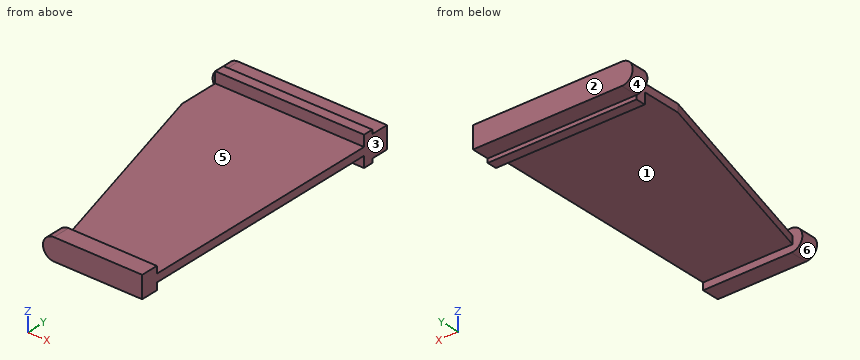
from build123d import *

# Parameters (mm, degrees)
BOSS_EXTRUDE1_DEPTH = 2.000000064
BOSS_EXTRUDE2_DEPTH = 4.4958
BOSS_EXTRUDE3_DEPTH = 4.4958
SKETCH4_W           = 38.1
SKETCH4_H           = 7.62
BOSS_EXTRUDE4_DEPTH = 2.54


with BuildPart() as part:
    # Sketch1 → Boss-Extrude1 (new body)
    with BuildSketch(Plane.XY):
        Polygon((0, 0), (-22.86, 0), (-38.1, 53.34), (-38.1, 66.04), (0, 66.04), align=None)
    extrude(amount=BOSS_EXTRUDE1_DEPTH)

    # Sketch2 → Boss-Extrude2 (add)
    with BuildSketch(Plane.XZ):
        with BuildLine():
            Line((0, -1.793999968), (-22.606, -1.793999968))
            ThreePointArc((-22.606, -1.793999968), (-25.4, 1.000000032), (-22.606, 3.794000032))
            Line((-22.606, 3.794000032), (0, 3.794000032))
            Line((0, 3.794000032), (0, -1.793999968))
        make_face()
    extrude(amount=BOSS_EXTRUDE2_DEPTH)

    # Sketch3 → Boss-Extrude3 (add)
    with BuildSketch(Plane(origin=(0, 66.04, 0), x_dir=(1, 0, 0), z_dir=(0, 1, 0))):
        with BuildLine():
            Line((0, 1.793999968), (0, -3.794000032))
            Line((0, -3.794000032), (-38.1, -3.794000032))
            ThreePointArc((-38.1, -3.794000032), (-40.894, -1.000000032), (-38.1, 1.793999968))
            Line((-38.1, 1.793999968), (0, 1.793999968))
        make_face()
    extrude(amount=BOSS_EXTRUDE3_DEPTH)

    # Sketch4 → Boss-Extrude4 (add)
    with BuildSketch(Plane.XZ.offset(-66.04)):
        with Locations((-19.05, 1.000000032)):
            Rectangle(SKETCH4_W, SKETCH4_H)
    extrude(amount=BOSS_EXTRUDE4_DEPTH)


solid = part.part
The model under review builds one solid part; all positions refer to its coordinate system, in mm. Face numbers are marked on the shaded views. A direction names the side the tool comes from. Coordinates: 2 decimals unless noted, no trailing zeros. Loops run counter-clockwise (first coordinate to the right, second up) from the corner with the lowest first, then second, coordinate; pieces in that order, holes last.
(1) Insertion check: P1, Ø3.5, axis at x = -27, y = 67.5, coming from the -Z side; P2, Ø2, axis at x = -40, z = 0, coming from the -Y side; P3, Ø1, axis at y = 6, z = 3, coming from the -X side; P4, Ø2, axis at x = -19.5, y = 67.5, coming from the +Z side. Each pin has a flat end and moves straight along its axis. Give the tip position at first contact, or say it passes through.
Determined:
P1: stops at z = -2.81
P2: stops at y = 66.04
P3: passes through
P4: stops at z = 3.79
(2) Consider section B-B, the plane z = 1. Give the boundary of the cut face in (x, y).
Determined:
outline: (-40.89, 66.04) - (-38.1, 66.04) - (-38.1, 53.34) - (-22.86, 0) - (-25.4, 0) - (-25.4, -4.5) - (0, -4.5) - (0, 70.54) - (-40.89, 70.54) - close
(3) Tool access review of the marked faces 4, 5 and 6: name each direction out of +Z, -Z, +X, -X, +Y, -Y from which nothing blocks a thin tool from reaching the whole face with its end or side.
Determined:
face 4: -X, +Y, -Y
face 5: +Z, +X, -X
face 6: -X, -Y
(4) Consider section D-D, the plane y = 51. Give the boundary of the cut face in (x, z).
Determined:
outline: (-37.43, 0) - (0, 0) - (0, 2) - (-37.43, 2) - close
(5) Draft analysis for pull direction Y (two halves, no side actions). For the marked faces 1, 2 and 3, state which applies: +Y half, -Y half, draft (parallel to the pull), parting line (faces both ways), or undercut.
Determined:
face 1: undercut
face 2: +Y half
face 3: draft
(6) Wall thickness on L1, parallel to Y at x = -10, z = 3; L2, parallel to Z at x = -7.5, y = 32; L3, parallel to Y at x = -35, z = -0.5: over which ranges is each line inside the solid? List them lowest first.
Determined:
L1: y = -4.5 to 0, 63.5 to 70.54
L2: z = 0 to 2
L3: y = 63.5 to 70.54
(7) Consider section A-A, the plane x = -19.5. Give the boundary of the cut face in (y, z), plus the area to 3 significant figures.
Determined:
outline: (-4.5, -1.79) - (0, -1.79) - (0, 0) - (63.5, 0) - (63.5, -2.81) - (66.04, -2.81) - (66.04, -1.79) - (70.54, -1.79) - (70.54, 3.79) - (66.04, 3.79) - (66.04, 4.81) - (63.5, 4.81) - (63.5, 2) - (0, 2) - (0, 3.79) - (-4.5, 3.79) - close
area: 197 mm2
(8) Consider section C-C, the plane y = 21. Give the boundary of the cut face in (x, z), plus the area to 3 significant figures.
Determined:
outline: (-28.86, 0) - (0, 0) - (0, 2) - (-28.86, 2) - close
area: 57.7 mm2
